from build123d import *

# Parameters (mm, degrees)
SALIENTE_EXTRUIR1_DEPTH = 8
CROQUIS2_R              = 4.25
SALIENTE_EXTRUIR2_DEPTH = 80
CROQUIS4_R              = 1.5
CORTAR_EXTRUIR1_DEPTH   = 5
CROQUIS5_R              = 1.5
CORTAR_EXTRUIR2_DEPTH   = 7
SALIENTE_EXTRUIR3_START = -70
CROQUIS6_R              = 7.5
CROQUIS6_R_2            = 4.25
SALIENTE_EXTRUIR3_DEPTH = 70
CROQUIS7_R              = 1.5
CORTAR_EXTRUIR3_DEPTH   = 10
CROQUIS11_R             = 2.5
CORTAR_EXTRUIR4_DEPTH   = 1.8


with BuildPart() as part:
    # Croquis1 → Saliente-Extruir1 (new body)
    with BuildSketch(Plane(origin=(0, 0, 0), x_dir=(-1, 0, 0), z_dir=(0, 0, -1))):
        Polygon((-5.547383556, 27.615747118), (-5.547383556, 26.030607477), (0.077616444, 23.983274909), (0.077616444, 21.809098061), (-5.547383556, 19.761765493), (-5.547383556, 18.176625852), (0.077616444, 16.129293284), (0.077616444, 13.955116436), (-5.547383556, 11.907783868), (-5.547383556, 10.322644227), (0.077616444, 8.275311659), (0.077616444, 6.101134811), (-5.547383556, 4.053802243), (-5.547383556, 2.468662602), (0.077616444, 0.421330034), (0.077616444, -1.752846814), (-5.547383556, -3.800179382), (-5.547383556, -5.385319023), (0.077616444, -7.432651591), (0.077616444, -9.606828439), (-5.547383556, -11.654161007), (-5.547383556, -13.239300648), (0.077616444, -15.286633216), (0.077616444, -17.460810064), (-5.547383556, -19.508142632), (-5.547383556, -21.093282273), (0.077616444, -23.140614841), (0.077616444, -25.314791689), (-5.547383556, -27.362124257), (-5.547383556, -28.947263898), (0.077616444, -30.994596466), (0.077616444, -32.08168489), (4.952616444, -32.08168489), (4.952616444, 27.91831511), (-4.71608483, 27.91831511), align=None)
    extrude(amount=-SALIENTE_EXTRUIR1_DEPTH)

    # Croquis2 → Saliente-Extruir2 (add)
    with BuildSketch(Plane(origin=(0, 27.91831511, 0), x_dir=(1, 0, 0), z_dir=(0, 1, 0))):
        with BuildLine():
            Line((-4.952616444, -8), (-4.952616444, -4))
            Line((-4.952616444, -4), (-4.952616444, 0))
            Line((-4.952616444, 0), (-3.691152355, 0))
            ThreePointArc((-3.691152355, 0), (-17.535441126, -4), (-3.691152355, -8))
            Line((-3.691152355, -8), (-4.952616444, -8))
        make_face()
        with Locations(Location((-10.035441126, -4, 0), (0, 0, 270))):
            Circle(CROQUIS2_R, mode=Mode.SUBTRACT)
    extrude(amount=-SALIENTE_EXTRUIR2_DEPTH)

    # Croquis4 → Cortar-Extruir1 (cut)
    with BuildSketch(Plane.ZY.offset(17.535441126)):
        with Locations((4, 12.91831511)):
            Circle(CROQUIS4_R)
        with Locations((4, -37.08168489)):
            Circle(CROQUIS4_R)
    extrude(amount=-CORTAR_EXTRUIR1_DEPTH, mode=Mode.SUBTRACT)

    # Croquis5 → Cortar-Extruir2 (cut, symmetric)
    with BuildSketch(Plane.ZY.offset(17.535441126)):
        with Locations(Location((4, -12.08168489, 0), (0, 0, 180))):
            Circle(CROQUIS5_R)
    extrude(amount=CORTAR_EXTRUIR2_DEPTH, both=True, mode=Mode.SUBTRACT)

    # Croquis6 → Saliente-Extruir3 (add)
    with BuildSketch(Plane.XZ.offset(52.08168489).offset(SALIENTE_EXTRUIR3_START)):
        with Locations(Location((-10.035441126, 4, 0), (0, 0, 90))):
            Circle(CROQUIS6_R)
        with Locations(Location((-10.035441126, 4, 0), (0, 0, 90))):
            Circle(CROQUIS6_R_2, mode=Mode.SUBTRACT)
    extrude(amount=SALIENTE_EXTRUIR3_DEPTH)

    # Croquis7 → Cortar-Extruir3 (cut)
    with BuildSketch(Plane.ZY.offset(17.535441126)):
        with Locations((4, -12.08168489)):
            Circle(CROQUIS7_R)
        with Locations((4, -37.08168489)):
            Circle(CROQUIS7_R)
        with Locations((4, 12.91831511)):
            Circle(CROQUIS7_R)
    extrude(amount=-CORTAR_EXTRUIR3_DEPTH, mode=Mode.SUBTRACT)

    # Croquis11 → Cortar-Extruir4 (cut)
    with BuildSketch(Plane.ZY.offset(17.535441126)):
        with Locations((4, 12.91831511)):
            Circle(CROQUIS11_R)
        with Locations((4, -12.08168489)):
            Circle(CROQUIS11_R)
        with Locations((4, -37.08168489)):
            Circle(CROQUIS11_R)
    extrude(amount=-CORTAR_EXTRUIR4_DEPTH, mode=Mode.SUBTRACT)


solid = part.part
Design review of the part built by this model. Coordinates are the model's own, in mm. A direction names the side the tool comes from. Coordinates: 2 decimals unless noted, no trailing zeros. Order: outer loops, then holes, each group sorted by start corner. A loop starts at its lowest first (then second) coordinate and runs counter-clockwise, first axis right, second up. Notation, with made-up numbers: (58.25, 88) -> (113.25, 88) arc R27 ccw to (113.25, 111) -> close; hole circle Ø2 at (-37, -33). An arc over 180 degrees is marked (long way). Use one line per item in the form item = value. Start each with the question number.
(1) Add section A-A on x = -10.75. State the section outline as (y, z) points.
(2) Insertion check: pin 1 (3 mm diameter, centred on y = 0.5, z = 8, fed in from -X); pin 2 (0.7 mm diameter, centred on y = -24, z = 4, fed in from +X); pin 3 (4.5 mm diameter, centred on x = -1, y = 2.5, fed in from +Z). Each pin has a flat end and moves straight along its axis. Give the tip position at first contact, or say it passes through.
(3) Add section D-D on z = 9.25. State the section outline as (x, y) points, plus the area to 3 significant figures.
(4) Add section B-B on z = 4. Give the number of separate pieces and of enclosed holes in the cut face, plus the area to 3 significant figures.
(5) For probe 1 along Y at (x, z) = (-16.75, 4); probe 2 along X at (y, z) = (-35.5, 4); probe 3 along Z at (x, y) = (-12.75, -32.5), list the stretches that pass through material, from the lowest coordinate up.
(6) The part is to be moulded in two halves that separate along Z. For faces 4 (the flat face through (-0.078, -24, 4)), 5 (the flat face through (-15.735, -12, 6)), say which applies: +Z half, -Z half, draft (parallel to the pull), parting line (faces both ways), or undercut.
(7) For faces 1 (the cylindrical face through (-16.4, -37, 1.5)), 2 (the flat face through (5.547, 19, 4)), 3 (the flat face through (-0.078, 15, 4)), list the 3-axis set-ups (+Z, -Z, +X, -X, +Y, -Y) from which the entire face can be reached by the end or side of a thin tool; tool diameter is ignored.
(8) Add section C-C on z = -1.5. State the section outline as (x, y) points.
Answer block:
q1.outline = (-52.08, -3.47) -> (27.92, -3.47) -> (27.92, -0.19) -> (-52.08, -0.19) -> close; (-52.08, 8.19) -> (27.92, 8.19) -> (27.92, 11.47) -> (-52.08, 11.47) -> close
q2.pin_1 = -17.11
q2.pin_2 = -0.08
q2.pin_3 = 8
q3.outline = (-15.39, -52.08) -> (-4.68, -52.08) -> (-4.68, 27.92) -> (-15.39, 27.92) -> close
q3.area = 857 mm²
q4.separate_pieces = 5
q4.enclosed_holes = 0
q4.area = 787 mm²
q5.probe_1 = -52.08 to -39.58, -34.58 to -14.58, -9.58 to 10.42, 15.42 to 27.92
q5.probe_2 = -15.74 to -14.29, -5.79 to -2.54
q5.probe_3 = -2.99 to 0.73, 7.27 to 10.99
q6.face_4 = draft
q6.face_5 = undercut
q7.face_1 = -X
q7.face_2 = +Z, -Z, +X, +Y, -Y
q7.face_3 = +Z, -Z, +X
q8.outline = (-15.13, -52.08) -> (-4.94, -52.08) -> (-4.94, 27.92) -> (-15.13, 27.92) -> close
